Here's how the part is built. I have some questions about the finished solid (model axes, mm). Face numbers are marked on the shaded views. Coordinates: 2 decimals unless noted, no trailing zeros. Write each loop counter-clockwise with the first axis right and the second up, starting at its lowest first coordinate (ties: lowest second). Pieces come first, ordered by that corner, then holes. Notation, with made-up numbers: (29.5, 86) -> (34.5, 86) arc R12 ccw to (34.5, 96) -> close; hole circle Ø7 at (87.25, 38.25). An arc over 180 degrees is marked (long way). Use a Markdown table: item, result. Add a question column.
Item 1: Imagine slicing it at A-A, the plane z = -1.5. Write out the boundary of the cut face in (x, y).
Item 2: If we mould it in two halves opening along X, with no side actions, what happens to the marked faces 1, 2 and 3? For each: pulls with the +X half, pulls with the -X half, needs draft (parallel to the pull), parting line crosses it, or undercut.
Item 3: Imagine slicing it at B-B, the plane x = -27.5. Write out the boundary of the cut face in (y, z).
Item 4: Will these pins go through, and if not, where does the flat tip stop? pin 1 Ø2 at (x, z) = (-13.5, 1) entering from +Y; pin 2 Ø3 at (x, z) = (-12.5, 0.5) entering from +Y; pin 3 Ø3 at (x, z) = (24.5, 0) entering from +Y.
Item 5: If I drill on line 1 along Y through (x, z) = (0, 1.4); line 2 along Y through (x, z) = (-26, -3); line 3 along Y through (x, z) = (10, 0.5), over which ranges is the centre line in solid material (lowest first)? Write a range as from..to.
Item 6: Imagine slicing it at C-C, the plane y = 22. Write out the boundary of the cut face in (x, z), and give its area (3 significant figures).
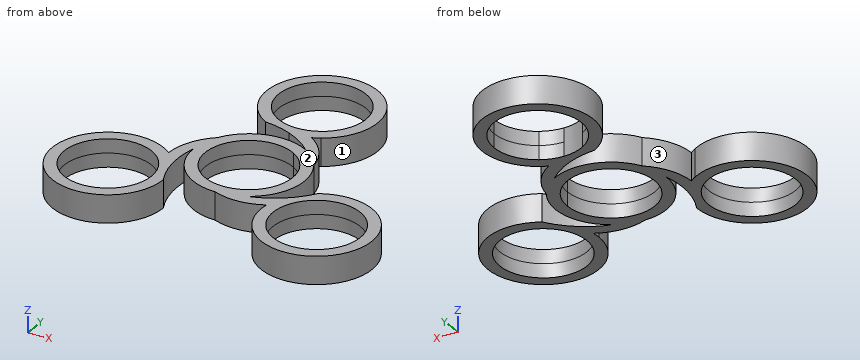
```python
from build123d import *

# Parameters (mm, degrees)
F0_R     = 11
F1_DEPTH = 3.5


# Not quite as in the source:
# - a feature of the source that left no trace in its solid (it failed there, or was rolled back) is left out


with BuildPart() as f1:
    # F0 (on Top) → F1 (new body, symmetric)
    with BuildSketch(Plane.XY):
        with BuildLine():
            ThreePointArc((9.5262794416, 5.5), (10.6251840892, 2.8470094961), (11, 0))
            ThreePointArc((11, 0), (-9.5262794416, -5.5), (5.5, 9.5262794416))
            Line((5.5, 9.5262794416), (7, 12.124355653))
            ThreePointArc((7, 12.124355653), (-3.6234666314, 13.522961568), (-12.124355653, 7))
            ThreePointArc((-12.124355653, 7), (-13.522961568, 3.6234666314), (-14, 0))
            ThreePointArc((-14, 0), (-13.522961568, -3.6234666314), (-12.124355653, -7))
            ThreePointArc((-12.124355653, -7), (-9.8994949366, -9.8994949366), (-7, -12.124355653))
            ThreePointArc((-7, -12.124355653), (-3.6234666314, -13.522961568), (0, -14))
            ThreePointArc((0, -14), (3.6234666314, -13.522961568), (7, -12.124355653))
            ThreePointArc((7, -12.124355653), (13.522961568, -3.6234666314), (12.124355653, 7))
            Line((12.124355653, 7), (9.5262794416, 5.5))
        make_face()
        with BuildLine():
            ThreePointArc((5.5, 9.5262794416), (7.7781745931, 7.7781745931), (9.5262794416, 5.5))
            Line((9.5262794416, 5.5), (12.124355653, 7))
            ThreePointArc((12.124355653, 7), (9.7975961228, 12.9972967743), (5.1726973399, 17.4685035196))
            ThreePointArc((5.1726973399, 17.4685035196), (6.1042077739, 17.8616349143), (7, 18.3304848581))
            ThreePointArc((7, 18.3304848581), (0, 44.4548405111), (-7, 18.3304848581))
            ThreePointArc((-7, 18.3304848581), (-3.4339564303, 17.8173408021), (0, 16.7274202555))
            ThreePointArc((0, 16.7274202555), (3.7217872887, 14.7631656496), (7, 12.124355653))
            Line((7, 12.124355653), (5.5, 9.5262794416))
        make_face()
        with BuildLine():
            ThreePointArc((5.5, 20.9285610695), (2.8470094961, 19.8296564219), (0, 19.4548405111))
            ThreePointArc((0, 19.4548405111), (-2.8470094961, 19.8296564219), (-5.5, 20.9285610695))
            ThreePointArc((-5.5, 20.9285610695), (-5.5, 39.9811199527), (11, 30.4548405111))
            ThreePointArc((11, 30.4548405111), (9.5262794416, 24.9548405111), (5.5, 20.9285610695))
        make_face(mode=Mode.SUBTRACT)
        with BuildLine():
            ThreePointArc((-14, 0), (-13.522961568, 3.6234666314), (-12.124355653, 7))
            ThreePointArc((-12.124355653, 7), (-16.1547872485, 1.9863187512), (-17.714516484, -4.2545644573))
            ThreePointArc((-17.714516484, -4.2545644573), (-18.5207334759, -3.644418455), (-19.3746655508, -3.1030646026))
            ThreePointArc((-19.3746655508, -3.1030646026), (-38.4990212038, -22.2274202555), (-12.3746655508, -15.2274202555))
            ThreePointArc((-12.3746655508, -15.2274202555), (-14.5592658851, -7.760146629), (-14, 0))
        make_face()
        with Locations((-26.3746655508, -15.2274202555)):
            Circle(F0_R, mode=Mode.SUBTRACT)
        with BuildLine():
            ThreePointArc((19.3746655508, -3.1030646026), (14.0001170604, -8.7286208024), (7, -12.124355653))
            ThreePointArc((7, -12.124355653), (3.6234666314, -13.522961568), (0, -14))
            ThreePointArc((0, -14), (6.3571911257, -14.9836155256), (12.5418191441, -13.2139390623))
            ThreePointArc((12.5418191441, -13.2139390623), (12.416525702, -14.2172164593), (12.3746655508, -15.2274202555))
            ThreePointArc((12.3746655508, -15.2274202555), (38.4990212038, -22.2274202555), (19.3746655508, -3.1030646026))
        make_face()
        with Locations((26.3746655508, -15.2274202555)):
            Circle(F0_R, mode=Mode.SUBTRACT)
    extrude(amount=F1_DEPTH, both=True)


solid = f1.part
```
Ans:
| question | item | result |
|---|---|---|
| 1 | outline | (-19.37, -3.1) arc R14 ccw (long way) to (-12.37, -15.23) arc R21.94 cw to (-14, 0) arc R14 ccw to (0, -14) arc R15 ccw to (12.54, -13.21) arc R12.21 ccw to (12.37, -15.23) arc R14 ccw (long way) to (19.37, -3.1) arc R21.94 cw to (7, -12.12) arc R14 ccw to (12.12, 7) arc R15 ccw to (5.17, 17.47) arc R12.21 ccw to (7, 18.33) arc R14 ccw (long way) to (-7, 18.33) arc R21.94 cw to (7, 12.12) arc R14 ccw to (-12.12, 7) arc R15 ccw to (-17.71, -4.25) arc R12.21 ccw to start; hole circle Ø22 at (-26.37, -15.23); hole circle Ø22 at (0, 0); hole circle Ø22 at (0, 30.45); hole circle Ø22 at (26.37, -15.23) |
| 2 | face 1 | parting line crosses it |
| 2 | face 2 | needs draft |
| 2 | face 3 | undercut |
| 3 | outline | (-29.18, -3.5) -> (-26.17, -3.5) -> (-26.17, 3.5) -> (-29.18, 3.5) -> close; (-4.29, -3.5) -> (-1.27, -3.5) -> (-1.27, 3.5) -> (-4.29, 3.5) -> close |
| 4 | pin 1 | stops at y = 36.76 |
| 4 | pin 2 | stops at y = 39.12 |
| 4 | pin 3 | stops at y = -1.23 |
| 5 | line 1 | y = -14..-11, 11..14, 16.73..19.45, 41.45..44.45 |
| 5 | line 2 | y = -29.22..-26.22, -4.23..-1.23 |
| 5 | line 3 | y = -14.3..-11.04, -9.8..-4.58, 4.58..12.68, 20.66..25.87, 35.04..40.25 |
| 6 | outline | (-11.16, -3.5) -> (-7.04, -3.5) -> (-7.04, 3.5) -> (-11.16, 3.5) -> close; (7.04, -3.5) -> (11.16, -3.5) -> (11.16, 3.5) -> (7.04, 3.5) -> close |
| 6 | area | 57.7 mm^2 |
